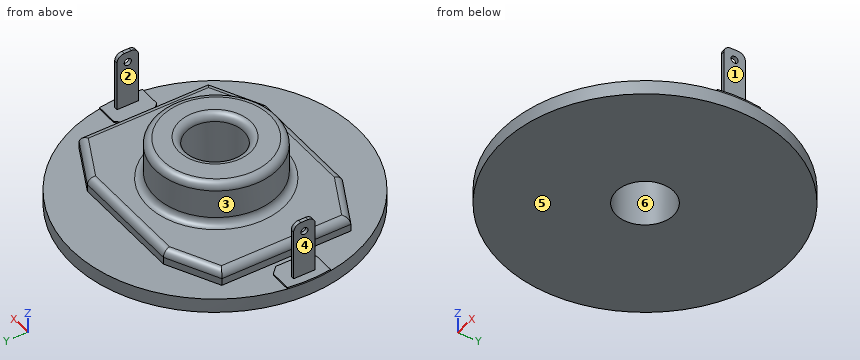
from build123d import *
from build123d.topology import SkipClean

# Parameters (mm, degrees)
BOSS_EXTRUDE1_DEPTH = 2
SKETCH2_R           = 20
BOSS_EXTRUDE2_DEPTH = 2
FILLET1_R           = 1
SKETCH3_R           = 8.5
BOSS_EXTRUDE3_DEPTH = 6
SKETCH4_R           = 4
CUT_EXTRUDE1_DEPTH  = 31
FILLET2_R           = 1
BOSS_EXTRUDE4_START = 0.2
BOSS_EXTRUDE4_DEPTH = 0.2
SKETCH6_W           = 0.5
SKETCH6_H           = 3
BOSS_EXTRUDE5_DEPTH = 8
FILLET3_R           = 1
SKETCH7_R           = 0.5
CUT_EXTRUDE2_DEPTH  = 4
CUT_EXTRUDE3_START  = -4
SKETCH8_R           = 0.5
CUT_EXTRUDE3_DEPTH  = 4


with BuildPart() as part:
    # Sketch1 → Boss-Extrude1 (new body)
    with BuildSketch(Plane.XY):
        Polygon((-15, 9), (-8, 12.5), (8, 12.5), (15, 9), (15, -9), (8, -12.5), (-8, -12.5), (-15, -9), align=None)
    extrude(amount=BOSS_EXTRUDE1_DEPTH)

    # Sketch2 → Boss-Extrude2 (add)
    with BuildSketch(Plane(origin=(0, 0, 0), x_dir=(-1, 0, 0), z_dir=(0, 0, -1))):
        Circle(SKETCH2_R)
    extrude(amount=BOSS_EXTRUDE2_DEPTH)

    # Fillet1
    fillet1_edges = [part.edges().sort_by_distance(p)[0] for p in [
        (-15, 0, 2),
        (-11.5, -10.75, 2),
        (0, -12.5, 2),
        (11.5, -10.75, 2),
        (15, 0, 2),
        (11.5, 10.75, 2),
        (0, 12.5, 2),
        (-11.5, 10.75, 2),
    ]]
    fillet(fillet1_edges, radius=FILLET1_R)

    # Sketch3 → Boss-Extrude3 (add)
    with BuildSketch(Plane.XY.offset(2)):
        with Locations(Location((-0.2660856, 0, 0), (0, 0, 180))):
            Circle(SKETCH3_R)
    extrude(amount=BOSS_EXTRUDE3_DEPTH)

    # Sketch4 → Cut-Extrude1 (cut, through all)
    with BuildSketch(Plane.XY.offset(8)):
        Circle(SKETCH4_R)
    extrude(amount=-CUT_EXTRUDE1_DEPTH, mode=Mode.SUBTRACT)

    # Fillet2
    fillet2_edges = [part.edges().sort_by_distance(p)[0] for p in [
        (8.2339144, 0, 2),
        (8.2339144, 0, 8),
        (-4, 0, 8),
    ]]
    fillet(fillet2_edges, radius=FILLET2_R)

    # Sketch5 → Boss-Extrude4 (add)
    with SkipClean():  # the faces are left unmerged after this step: merging them gives an invalid solid
        with BuildSketch(Plane.XY.offset(BOSS_EXTRUDE4_START)):
            with BuildLine():
                Line((-19.773719933, 3), (-16.773719933, 3))
                Line((-16.773719933, 3), (-15.773719933, 2))
                Line((-15.773719933, 2), (-15.773719933, -2))
                Line((-15.773719933, -2), (-16.773719933, -3))
                Line((-16.773719933, -3), (-19.773719933, -3))
                ThreePointArc((-19.773719933, -3), (-20, 0), (-19.773719933, 3))
            make_face()
            with BuildLine():
                Line((19.773719933, 3), (16.773719933, 3))
                Line((16.773719933, 3), (15.773719933, 2))
                Line((15.773719933, 2), (15.773719933, -2))
                Line((15.773719933, -2), (16.773719933, -3))
                Line((16.773719933, -3), (19.773719933, -3))
                ThreePointArc((19.773719933, -3), (20, 0), (19.773719933, 3))
            make_face()
        extrude(amount=-BOSS_EXTRUDE4_DEPTH)

    # Sketch6 → Boss-Extrude5 (add)
    with SkipClean():  # the faces are left unmerged after this step: merging them gives an invalid solid
        with BuildSketch(Plane.XY.offset(0.2)):
            with Locations((-18.564246067, 0.012841423)):
                Rectangle(SKETCH6_W, SKETCH6_H)
            with Locations((18.564246067, 0.012841423)):
                Rectangle(SKETCH6_W, SKETCH6_H)
        extrude(amount=BOSS_EXTRUDE5_DEPTH)

    # Fillet3
    fillet3_edges = [part.edges().sort_by_distance(p)[0] for p in [
        (-18.564246067, 1.512841423, 8.2),
        (-18.564246067, -1.487158577, 8.2),
        (18.564246067, 1.512841423, 8.2),
        (18.564246067, -1.487158577, 8.2),
    ]]
    fillet(fillet3_edges, radius=FILLET3_R)

    # Sketch7 → Cut-Extrude2 (cut)
    with BuildSketch(Plane.ZY.offset(18.814246067)):
        with Locations((6.7, 0.012841423)):
            Circle(SKETCH7_R)
    extrude(amount=-CUT_EXTRUDE2_DEPTH, mode=Mode.SUBTRACT)

    # Sketch8 → Cut-Extrude3 (cut)
    with BuildSketch(Plane(origin=(18.814246067, 0, 0), x_dir=(0, 0, -1), z_dir=(1, 0, 0)).offset(CUT_EXTRUDE3_START)):
        with Locations(Location((-6.7, 0.012841423, 0), (0, 0, 180))):
            Circle(SKETCH8_R)
    extrude(amount=CUT_EXTRUDE3_DEPTH, mode=Mode.SUBTRACT)


solid = part.part
CAD build for the part. Positions are in the model's coordinates, mm. Face numbers are marked on the shaded views. A direction names the side the tool comes from. Coordinates: 2 decimals unless noted, no trailing zeros. Write each loop counter-clockwise with the first axis right and the second up, starting at its lowest first coordinate (ties: lowest second). Pieces come first, ordered by that corner, then holes. Notation, with made-up numbers: (-27, 83) - (24, 83) arc R36 ccw to (24, 120) - close; hole circle Ø4 at (56.5, 9). An arc over 180 degrees is marked (long way). Use a Markdown table: item, result. Add a question column.
Item 1: Flat gauge pins, fed straight in: pin 1 (1.1 mm diameter, centred on x = 0, z = 0.5, fed in from +Y); pin 2 (1.1 mm diameter, centred on y = -3, z = 0.5, fed in from -X); pin 3 (1 mm diameter, centred on x = 1, y = 4.5, fed in from +Z). Where does each tip first touch, or does it go through?
Item 2: Drill centre lines: L1, parallel to Y at x = -18.5, z = 6.7; L2, parallel to Z at x = 8, y = -7; L3, parallel to Z at x = -6, y = 13. Where is each one in solid material? Low to high. Write a range as from..to.
Item 3: 3-axis set-ups, long thin cutter, end or side, ignore diameter. For the marked faces 1, 2 and 3: which of +Z, -Z, +X, -X, +Y, -Y reach the whole face in a straight line?
Item 4: Band-saw the part on A-A, the plane z = 3.75. Give the cut face in (x, y).
Item 5: Mould opens along X. For the marked faces 4, 5 and 6 say: pulls with the +X half, pulls with the -X half, needs draft (parallel to the pull), parting line crosses it, or undercut.
Numbers:
| question | item | result |
|---|---|---|
| 1 | pin 1 | y = 20 |
| 1 | pin 2 | x = -19.84 |
| 1 | pin 3 | z = 8 |
| 2 | L1 | -1.49..-0.49, 0.51..1.51 |
| 2 | L2 | -2..2 |
| 2 | L3 | -2..0 |
| 3 | face 1 | +Z, +X, +Y, -Y |
| 3 | face 2 | +Z, +Y, -Y |
| 3 | face 3 | +Z |
| 4 | outline | (-18.81, -1.49) - (-18.31, -1.49) - (-18.31, 1.51) - (-18.81, 1.51) - close; circle Ø17 at (-0.27, 0); (18.31, -1.49) - (18.81, -1.49) - (18.81, 1.51) - (18.31, 1.51) - close; hole circle Ø8 at (0, 0) |
| 5 | face 4 | pulls with the -X half |
| 5 | face 5 | needs draft |
| 5 | face 6 | undercut |
